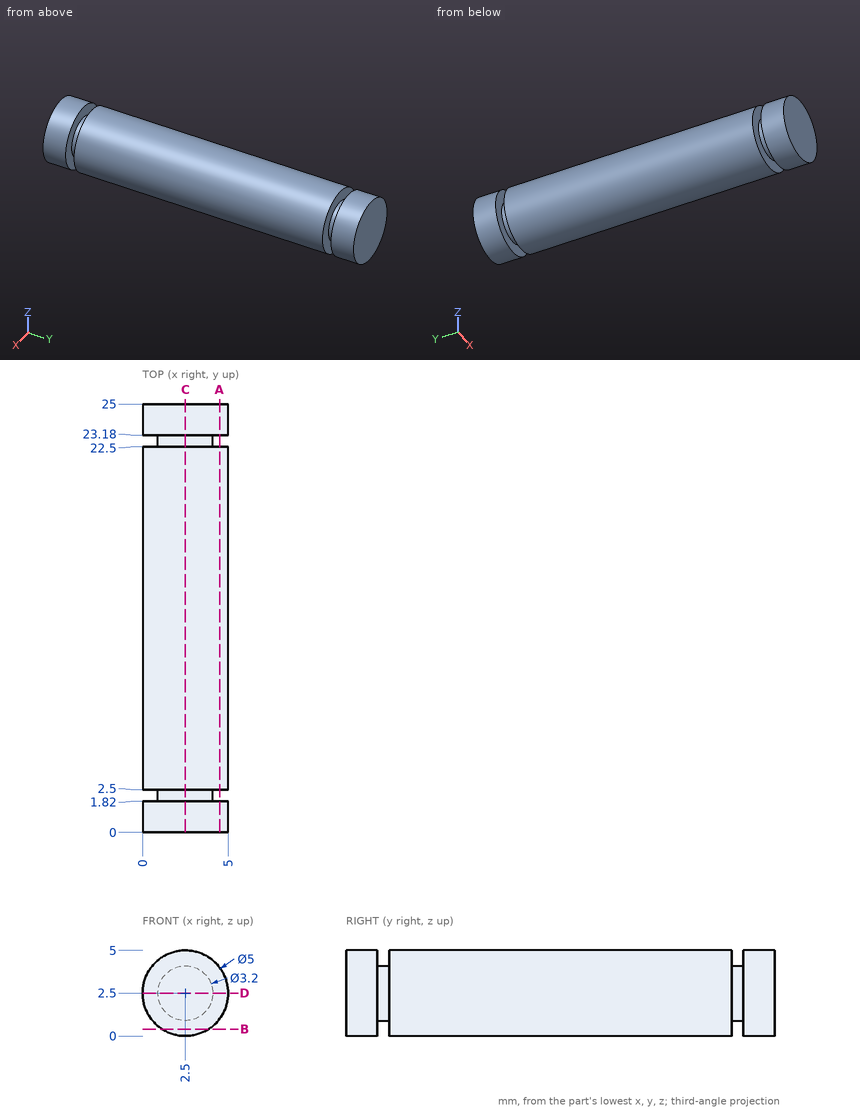
Here's the drawing with two shaded views (mm, measured from the low corner). I have some questions. Coordinates: 2 decimals unless noted, no trailing zeros. Order: outer loops, then holes, each group sorted by start corner. A loop starts at its lowest first (then second) coordinate and runs counter-clockwise, first axis right, second up. Notation, with made-up numbers: (79, -19) - (102, -19) arc R29 ccw to (102, 16) - close; hole circle Ø9 at (83, 36). An arc over 180 degrees is marked (long way). Answer in a Markdown table with one row per item.
1. Suppose I cut it at D-D (z = 2.5). Please give me the cut outline in (x, y).
Reply:
| item | result |
|---|---|
| outline | (0, 0) - (5, 0) - (5, 1.82) - (4.1, 1.82) - (4.1, 2.5) - (5, 2.5) - (5, 22.5) - (4.1, 22.5) - (4.1, 23.18) - (5, 23.18) - (5, 25) - (0, 25) - (0, 23.18) - (0.9, 23.18) - (0.9, 22.5) - (0, 22.5) - (0, 2.5) - (0.9, 2.5) - (0.9, 1.82) - (0, 1.82) - close |
2. Suppose I cut it at A-A (x = 4.5). Please give me the cut outline in (y, z).
Reply:
| item | result |
|---|---|
| outline | (0, 1) - (1.82, 1) - (1.82, 4) - (0, 4) - close; (2.5, 1) - (22.5, 1) - (22.5, 4) - (2.5, 4) - close; (23.18, 1) - (25, 1) - (25, 4) - (23.18, 4) - close |
3. For pin 1 (1 mm diameter, centred on x = 1.5, y = 6, fed in from -Z); pin 2 (1 mm diameter, centred on y = 11.5, z = 3, fed in from +X), each with a flat end and sliding along its axis, tell me the tip position at first contact or that it passes through.
Reply:
| item | result |
|---|---|
| pin 1 | stops at z = 0.05 |
| pin 2 | stops at x = 5 |
4. If I drill on line 1 along Y through (x, z) = (0.65, 3.45); line 2 along X through (y, z) = (10.25, 3.45); line 3 along X through (y, z) = (5.5, 1.2), over which ranges is the centre line in solid material (lowest first)?
Reply:
| item | result |
|---|---|
| line 1 | y = 0 to 1.82, 2.5 to 22.5, 23.18 to 25 |
| line 2 | x = 0.19 to 4.81 |
| line 3 | x = 0.36 to 4.64 |
5. Suppose I cut it at B-B (z = 0.4). Please give me the cut outline in (x, y), and give its area (3 significant figures).
Reply:
| item | result |
|---|---|
| outline | (1.14, 0) - (3.86, 0) - (3.86, 1.82) - (1.14, 1.82) - close; (1.14, 2.5) - (3.86, 2.5) - (3.86, 22.5) - (1.14, 22.5) - close; (1.14, 23.18) - (3.86, 23.18) - (3.86, 25) - (1.14, 25) - close |
| area | 64.1 mm^2 |
6. Suppose I cut it at C-C (x = 2.5). Please give me the cut outline in (y, z).
Reply:
| item | result |
|---|---|
| outline | (0, 0) - (1.82, 0) - (1.82, 0.9) - (2.5, 0.9) - (2.5, 0) - (22.5, 0) - (22.5, 0.9) - (23.18, 0.9) - (23.18, 0) - (25, 0) - (25, 5) - (23.18, 5) - (23.18, 4.1) - (22.5, 4.1) - (22.5, 5) - (2.5, 5) - (2.5, 4.1) - (1.82, 4.1) - (1.82, 5) - (0, 5) - close |
